Design review of the part built by this model. Coordinates are the model's own, in mm. Face numbers are marked on the shaded views. A direction names the side the tool comes from. Coordinates: 2 decimals unless noted, no trailing zeros. Loops run counter-clockwise (first coordinate to the right, second up) from the corner with the lowest first, then second, coordinate; pieces in that order, holes last. Notation, with made-up numbers: (-9, 40) -> (16, 40) arc R33 ccw to (16, 75) -> close; hole circle Ø10 at (33, -33.5). An arc over 180 degrees is marked (long way). Use one line per item in the form item = value. Start each with the question number.
1. Machinability: for the marked faces 5 and 6, which of the approach directions +Z, -Z, +X, -X, +Y, -Y give a long, thin tool a straight path to every point of the face, cutting with its end or side? Answer none if there is none.
2. For pin 1 (2 mm diameter, centred on x = 5, z = 6, fed in from +Y); pin 2 (4 mm diameter, centred on x = -1.5, y = 4.5, fed in from +Z), all flat-tipped, find the tip position at first contact; note any pin that passes through.
3. Consider section C-C (z = -12.5). State the section outline as (x, y) points (3 decimals), then the cut area to 3 significant figures.
4. Consider section A-A (z = 40). State the section outline as (x, y) points, then the cut area to 3 significant figures.
5. The part is to be moulded in two halves that separate along X. For the marked faces 1, 2, 3 and 4, say which applies: released by +X, released by -X, zero draft, split by the parting line, or undercut.
6. Consider section B-B (y = 4). State how many separate pieces and enclosed holes the cut face has, then the cut area to 3 significant figures.
7. Wall thickness on line 1 (Y direction, x = 10, z = 40); line 2 (X direction, y = 0.5, z = 23); line 3 (X direction, y = 4.75, z = 34): over which ranges is each line inside the solid? List them lowest first. Write a range as from..to.
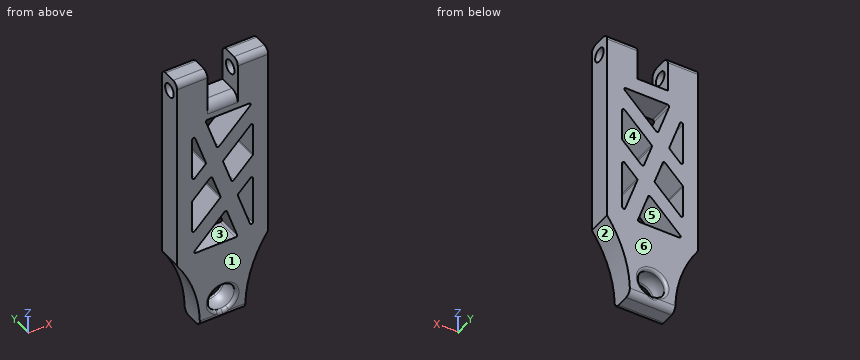
from build123d import *

# Parameters (mm, degrees)
SKETCH1_W               = 30
SKETCH1_H               = 90
BOSS_EXTRUDE1_DEPTH     = 8
SKETCH2_W               = 10
SKETCH2_H               = 12
CUT_EXTRUDE1_DEPTH      = 8
SKETCH3_R               = 2.25
CUT_EXTRUDE2_DEPTH      = 55.671747731
FILLET1_R               = 2
CUT_EXTRUDE3_DEPTH      = 49.104053883
FILLET2_R               = 3
FILLET3_R               = 0.9
CUT_EXTRUDE4_DEPTH      = 49.104054025
CUT_EXTRUDE4_DEPTH_BACK = 49.104054025
FILLET4_R               = 0.5


with BuildPart() as part:
    # Sketch1 → Boss-Extrude1 (new body)
    with BuildSketch(Plane(origin=(0, 0, 0), x_dir=(1, 0, 0), z_dir=(0, 1, 0))):
        Rectangle(SKETCH1_W, SKETCH1_H)
    extrude(amount=BOSS_EXTRUDE1_DEPTH)

    # Sketch2 → Cut-Extrude1 (cut)
    with BuildSketch(Plane(origin=(0, 8, 0), x_dir=(1, 0, 0), z_dir=(0, 1, 0))):
        with Locations((0, -39)):
            Rectangle(SKETCH2_W, SKETCH2_H)
    extrude(amount=-CUT_EXTRUDE1_DEPTH, mode=Mode.SUBTRACT)

    # Sketch3 → Cut-Extrude2 (cut, through all)
    with BuildSketch(Plane(origin=(15, 0, 0), x_dir=(0, 0, -1), z_dir=(1, 0, 0))):
        with Locations((-40, 4)):
            Circle(SKETCH3_R)
    extrude(amount=-CUT_EXTRUDE2_DEPTH, mode=Mode.SUBTRACT)

    # Fillet1
    fillet1_edges = [part.edges().sort_by_distance(p)[0] for p in [
        (10, 0, 45),
        (-10, 8, 45),
        (10, 8, 45),
        (-10, 0, 45),
        (0, 0, -45),
        (0, 8, -45),
    ]]
    fillet(fillet1_edges, radius=FILLET1_R)

    # Sketch4 → Cut-Extrude3 (cut, through all)
    with BuildSketch(Plane(origin=(0, 8, 0), x_dir=(1, 0, 0), z_dir=(0, 1, 0))):
        Polygon((5, 18), (-10, 18), (1.186440678, 6.813559322), align=None)
        Polygon((10, -2), (10, 18), (4.915254237, 3.084745763), align=None)
        Polygon((-10, -8), (-10, -26), (-5.423728814, -12.576271186), align=None)
        Polygon((-5.681818182, -28), (10, -28), (-1.694915254, -16.305084746), align=None)
        Polygon((-10, 10.928932188), (-10, -0.928932188), (-3.625999709, -7.302932479), (-0.611288427, 1.540220615), align=None)
        Polygon((10.002308787, -20.931240975), (10.002308787, -9.073376599), (3.117525133, -2.188592944), (0.10281385, -11.031746039), align=None)
    extrude(amount=-CUT_EXTRUDE3_DEPTH, mode=Mode.SUBTRACT)

    # Fillet2
    fillet2_edges = [part.edges().sort_by_distance(p)[0] for p in [
        (0, 0, 33),
    ]]
    fillet(fillet2_edges, radius=FILLET2_R)

    # Sketch5 → Cut-Revolve1 (revolve, cut)
    with BuildSketch(Plane(origin=(0, 0, 0), x_dir=(0, 0, -1), z_dir=(1, 0, 0))):
        with BuildLine():
            Line((41.5, 8), (38, 8))
            Line((38, 8), (38, 0))
            Line((38, 0), (41.5, 0))
            ThreePointArc((41.5, 0), (43.315072906, 4), (41.5, 8))
        make_face()
    revolve(axis=Axis((0, 8, -38), (0, -1, 0)), mode=Mode.SUBTRACT)

    # Fillet3
    fillet3_edges = [part.edges().sort_by_distance(p)[0] for p in [
        (0, 0, -34.5),
        (0, 8, -34.5),
    ]]
    fillet(fillet3_edges, radius=FILLET3_R - 0.0004)  # a hair under: the kernel refuses the full size

    # Sketch6 → Cut-Extrude4 (cut, two sides: drawn at the far end of the back side and taken through both)
    with BuildSketch(Plane(origin=(0, 8, 0), x_dir=(1, 0, 0), z_dir=(0, 1, 0)).offset(-CUT_EXTRUDE4_DEPTH_BACK)):
        with BuildLine():
            Line((-7.477541934, 45), (-15, 45))
            Line((-15, 45), (-15, 20.080818258))
            ThreePointArc((-15, 20.080818258), (-9.275408523, 31.947720661), (-7.477541934, 45))
        make_face()
        with BuildLine():
            Line((15, 45), (15, 20.080818258))
            ThreePointArc((15, 20.080818258), (9.275408523, 31.947720661), (7.477541934, 45))
            Line((7.477541934, 45), (15, 45))
        make_face()
    extrude(amount=CUT_EXTRUDE4_DEPTH + CUT_EXTRUDE4_DEPTH_BACK, mode=Mode.SUBTRACT)

    # Fillet4
    fillet4_edges = [part.edges().sort_by_distance(p)[0] for p in [
        (-10, 4, -10.928932188),
        (-0.611288427, 4, -1.540220615),
        (-3.625999709, 4, 7.302932479),
        (-10, 4, 0.928932188),
        (-1.694915254, 4, 16.305084746),
        (10, 4, 28),
        (-5.681818182, 4, 28),
        (10, 4, 2),
        (4.915254237, 4, -3.084745763),
        (10, 4, -18),
        (-10, 4, 8),
        (-5.423728814, 4, 12.576271186),
        (-10, 4, 26),
        (10.002308787, 4, 20.931240975),
        (0.10281385, 4, 11.031746039),
        (3.117525133, 4, 2.188592944),
        (10.002308787, 4, 9.073376599),
        (5, 4, -18),
        (1.186440678, 4, -6.813559322),
        (-10, 4, -18),
    ]]
    fillet(fillet4_edges, radius=FILLET4_R)


solid = part.part
Geometry check:
q1.face_5 = +Y, -Y
q1.face_6 = +Z, -Z, +X, -X, +Y
q2.pin_1 = through
q2.pin_2 = 33
q3.outline = (-15, 0) -> (-4.5, 0) -> (-4.5, 8) -> (-15, 8) -> close; (3.125, 0) -> (8.125, 0) -> (8.125, 8) -> (3.125, 8) -> close; (10, 0) -> (15, 0) -> (15, 8) -> (10, 8) -> close
q3.area = 164 mm²
q4.outline = (-15, 0) -> (-5, 0) -> (-5, 1.75) -> (-15, 1.75) -> close; (-15, 6.25) -> (-5, 6.25) -> (-5, 8) -> (-15, 8) -> close; (5, 0) -> (15, 0) -> (15, 1.75) -> (5, 1.75) -> close; (5, 6.25) -> (15, 6.25) -> (15, 8) -> (5, 8) -> close
q4.area = 70.0 mm²
q5.face_1 = zero draft
q5.face_2 = released by +X
q5.face_3 = undercut
q5.face_4 = undercut
q6.separate_pieces = 3
q6.enclosed_holes = 7
q6.area = 1,690 mm²
q7.line_1 = 0..1.75, 6.25..8
q7.line_2 = -15..-10, -8.98..-3.98, 5..15
q7.line_3 = -15..-5, 5..15
